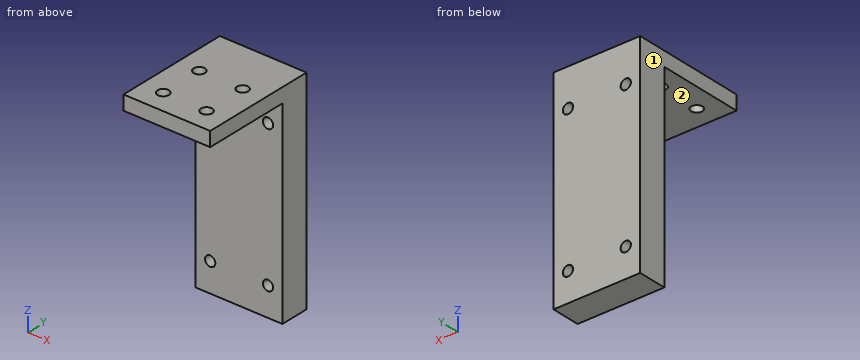
Autodesk Inventor part; units mm, degrees
ref_plane "YZ Plane" through (0, 0, 0) normal (1, 0, 0) x (0, 1, 0)
ref_plane "XZ Plane" through (0, 0, 0) normal (0, 1, 0) x (-1, 0, 0)
ref_plane "XY Plane" through (0, 0, 0) normal (0, 0, 1) x (1, 0, 0)
sketch "Sketch2" plane through (0, 0, 0) normal (0, 1, 0) x (-1, 0, 0)
  line L0 (-19.05, 44.45) -> (-19.05, -44.45)
  line L1 (-19.05, -44.45) -> (19.05, -44.45)
  line L2 (19.05, -44.45) -> (19.05, 44.45)
  line L3 (19.05, 44.45) -> (-19.05, 44.45) construction
  line L4 (-19.05, 44.45) -> (19.05, -44.45) construction
  line L5 (-19.05, -44.45) -> (19.05, 44.45) construction
  line L6 (19.05, 44.45) -> (19.05, 48.26)
  line L7 (19.05, 48.26) -> (-19.05, 48.26)
  line L8 (-19.05, 48.26) -> (-19.05, 43.3404)
  point P0 (0, 0)
  dimension "lengthBaseAirCylinder" = 88.9
  dimension "widthBaseOfAirCylinder" = 38.1
  dimension "extenstionForStroke" = 3.81
extrude "Extrusion1" add sketch "Sketch2" against normal blind 12.7
sketch "Sketch3" plane through (0, -12.7, 0) normal (0, -1, 0) x (1, 0, 0)
  line L0 (19.05, -44.45) -> (19.05, 48.26)
  line L1 (-19.05, 48.26) -> (-19.05, -44.45)
  line L2 (19.05, 48.26) -> (-19.05, 48.26)
  line L3 (-19.05, 48.26) -> (-19.05, 41.91)
  line L4 (-19.05, 41.91) -> (19.05, 41.91)
  line L5 (19.05, 41.91) -> (19.05, 48.26)
  point P0 (0, 0)
  dimension "d9" = 6.35
extrude "Extrusion2" add sketch "Sketch3" along normal blind 38.1
sketch "Sketch4" plane through (0, 0, 0) normal (0, 1, 0) x (1, 0, 0)
  line L0 (12.7, -31.75) -> (12.7, 31.75) construction
  line L1 (12.7, 31.75) -> (-12.7, 31.75) construction
  line L2 (-12.7, 31.75) -> (-12.7, -31.75) construction
  line L3 (-12.7, -31.75) -> (12.7, -31.75) construction
  line L4 (12.7, -31.75) -> (-12.7, 31.75) construction
  line L5 (12.7, 31.75) -> (-12.7, -31.75) construction
  point P0 (0, 0)
  dimension "widthForCylinderBoltHoles" = 25.4
  dimension "lengthForCylinderHoles" = 63.5
hole "Hole1" at (12.7, 0, 31.75) at (12.7, 0, -31.75) at (-12.7, 0, -31.75) at (-12.7, 0, 31.75) direction (0, -1, 0) diameter 4.4958 end through all
sketch "Sketch5" plane through (-19.05, 0, 48.26) normal (0, 0, 1) x (1, 0, 0)
  line L0 (38.1, -12.7) -> (0, -12.7)
  line L1 (19.05, -12.7) -> (19.05, -50.8) construction
  line L2 (38.1, -50.8) -> (0, -50.8) construction
  line L3 (9.525, -41.275) -> (28.575, -41.275) construction
  line L4 (28.575, -41.275) -> (28.575, -22.225) construction
  line L5 (28.575, -22.225) -> (9.525, -22.225) construction
  line L6 (9.525, -22.225) -> (9.525, -41.275) construction
  line L7 (9.525, -41.275) -> (28.575, -22.225) construction
  line L8 (28.575, -41.275) -> (9.525, -22.225) construction
  point P0 (19.05, 0)
  point P1 (19.05, -31.75)
  dimension "d21" = 19.05
  dimension "d22" = 19.05
hole "Hole2" at (-9.525, -41.275, 48.26) at (9.525, -41.275, 48.26) at (9.525, -22.225, 48.26) at (-9.525, -22.225, 48.26) direction (0, 0, -1) diameter 4.9784 end through all
properties part number "SupportForStopAirCylinder" material "Aluminum 6061"
Could you check a few things on this model? Use its own coordinates, in mm. Face numbers are marked on the shaded views. A direction names the side the tool comes from. Coordinates: 2 decimals unless noted, no trailing zeros. Write each loop counter-clockwise with the first axis right and the second up, starting at its lowest first coordinate (ties: lowest second). Pieces come first, ordered by that corner, then holes. Notation, with made-up numbers: (-17, 67.5) -> (25, 67.5) arc R20 cw to (25, 79.5) -> close; hole circle Ø11 at (45, 79). An arc over 180 degrees is marked (long way). Write item = value, one per line. Start each with the question number.
(1) I need wall thicknesses on line 1 (Z direction, x = 12.5, y = -12); line 2 (Z direction, x = 12, y = -6); line 3 (Y direction, x = 5, z = 12). Which ranges of each line are inside material? Lowest first, please. Write a range as [from, to].
(2) I want a section at B-B (x = -8). Please give me the cut outline in (y, z), plus the area to 3 significant figures.
(3) Will these pins go through, and if not, where does the flat tip stop? pin 1 (3 mm diameter, centred on x = 3.5, y = -27, fed in from -Z); pin 2 (4.5 mm diameter, centred on x = 9.525, y = -22.225, fed in from -Z); pin 3 (7 mm diameter, centred on x = 12.7, z = 31.75, fed in from -Y); pin 4 (12 mm diameter, centred on x = 11, y = -22, fed in from +Z).
(4) I want a section at A-A (z = 31.75). Please give me the cut outline in (x, y).
(5) Which directions (+Z, -Z, +X, -X, +Y, -Y) give clear straight access to the entire face, cutting with the end or side of a thin tool? Please do the marked faces 1 and 2.
(6) I want a section at D-D (z = -5). Please give me the cut outline in (x, y).
(7) I want a section at C-C (x = 3.5). Please give me the cut outline in (y, z), plus the area to 3 significant figures.
Result set:
q1.line_1 = [-44.45, -33.99], [-29.51, 29.51], [33.99, 48.26]
q1.line_2 = [-44.45, -33.89], [-29.61, 29.61], [33.89, 48.26]
q1.line_3 = [-12.7, 0]
q2.outline = (-50.8, 41.91) -> (-43.24, 41.91) -> (-43.24, 48.26) -> (-50.8, 48.26) -> close; (-39.31, 41.91) -> (-24.19, 41.91) -> (-24.19, 48.26) -> (-39.31, 48.26) -> close; (-20.26, 41.91) -> (-12.7, 41.91) -> (-12.7, -44.45) -> (0, -44.45) -> (0, 48.26) -> (-20.26, 48.26) -> close
q2.area = 1,370 mm2
q3.pin_1 = 41.91
q3.pin_2 = through
q3.pin_3 = -12.7
q3.pin_4 = 48.26
q4.outline = (-19.05, -12.7) -> (-14.95, -12.7) -> (-14.95, 0) -> (-19.05, 0) -> close; (-10.45, -12.7) -> (10.45, -12.7) -> (10.45, 0) -> (-10.45, 0) -> close; (14.95, -12.7) -> (19.05, -12.7) -> (19.05, 0) -> (14.95, 0) -> close
q5.face_1 = +Z, -Z, -X, +Y, -Y
q5.face_2 = -Z, +X, -X, -Y
q6.outline = (-19.05, -12.7) -> (19.05, -12.7) -> (19.05, 0) -> (-19.05, 0) -> close
q7.outline = (-50.8, 41.91) -> (-12.7, 41.91) -> (-12.7, -44.45) -> (0, -44.45) -> (0, 48.26) -> (-50.8, 48.26) -> close
q7.area = 1,420 mm2
